Here's how the part is built. I have some questions about the finished solid (model axes, mm). Face numbers are marked on the shaded views. A direction names the side the tool comes from. Coordinates: 2 decimals unless noted, no trailing zeros. Write each loop counter-clockwise with the first axis right and the second up, starting at its lowest first coordinate (ties: lowest second). Pieces come first, ordered by that corner, then holes. Notation, with made-up numbers: (34.25, -2.5) - (76.25, -2.5) arc R23 ccw to (76.25, 14.5) - close; hole circle Ø5 at (-6.5, 58). An arc over 180 degrees is marked (long way). Answer in a Markdown table with one row per item. Add a question column.
Item 1: Imagine slicing it at B-B (y = 11). Please give me the cut outline in (x, z), plus the area to 3 significant figures.
Item 2: We'd pull the mould along Z, two halves only. Please class the marked faces 1, 2 and 3: +Z half, -Z half, draft (parallel to the pull), parting line (faces both ways), or undercut.
Item 3: If I drill on probe 1 along X at (y, z) = (12, 6); probe 2 along X at (y, z) = (10, 6); probe 3 along Y at (x, z) = (-8, 7.5), over which ranges is the centre line in solid material (lowest first)? Write a range as from..to.
Item 4: Imagine slicing it at D-D (z = 2.75). Please give me the cut outline in (x, y).
Item 5: I'm going to push flat-ended pins straight in: pin 1 (12 mm diameter, centred on x = -36, y = -3.5, fed in from -Z); pin 2 (5.5 mm diameter, centred on x = 1.95, z = 6, fed in from -Y); pin 3 (2 mm diameter, centred on x = -21, z = 8.5, fed in from -Y). Where does each tip first touch, or does it pass through?
Item 6: Imagine slicing it at C-C (x = -16). Please give me the cut outline in (y, z).
Item 7: Imagine slicing it at A-A (z = 10). Please give me the cut outline in (x, y), plus the area to 3 significant figures.
Item 8: Which directions (+Z, -Z, +X, -X, +Y, -Y) give clear straight access to the entire face, cutting with the end or side of a thin tool? Please do the marked faces 4 and 5.
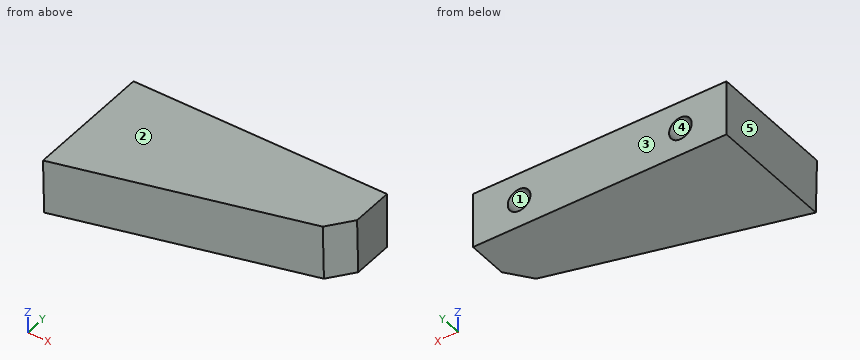
Autodesk Inventor part; units mm, degrees
ref_plane "作業平面8" through (7.9805, 5.1586, 3) normal (0.2539, -0.9668, -0.0285) x (-0.9522, -0.2551, 0.1679)
ref_plane "YZ Plane" through (0, 0, 0) normal (1, 0, 0) x (0, 1, 0)
ref_plane "XZ Plane" through (0, 0, 0) normal (0, 1, 0) x (-1, 0, 0)
sketch "スケッチ2" plane through (0, 0, 0) normal (0, 0, 1) x (1, 0, 0)
  line L0 (-43.0479, 19.0453) -> (-43.0479, -8.9547)
  line L1 (-43.0479, -8.9547) -> (11.9521, -8.9547)
  line L2 (11.9521, -8.9547) -> (11.9521, 19.0453)
  line L3 (11.9521, 19.0453) -> (-43.0479, 19.0453)
  point P0 (0, 0)
  dimension "d3" = 55
  dimension "d16" = 28
extrude "押し出し2" add sketch "スケッチ2" along normal blind 12
sketch "スケッチ4" plane through (-43.0479, 19.0453, 0) normal (0, 1, 0) x (1, 0, 0)
  line L0 (55, 0) -> (55, -12)
  line L1 (0, 0) -> (0, -12)
  line L2 (0, -6) -> (55, -6)
  line L3 (0, -12) -> (55, -12)
  line L4 (0, 0) -> (55, 0)
  point P0 (10, -6)
  point P1 (45, -6)
  dimension "d17" = 10
  dimension "d18" = 35
hole "穴2" at (-33.0479, 19.0453, 6) at (1.9521, 19.0453, 6) direction (0, -1, 0) diameter 4.917 depth 12 tip angle 118
ref_plane "作業平面8" through (7.9805, 5.1586, 3) normal (0.2539, -0.9668, -0.0285) x (-0.9522, -0.2551, 0.1679)
sketch "スケッチ7" plane through (7.9805, 5.1586, 3) normal (0.2539, -0.9668, -0.0285) x (-0.9522, -0.2551, 0.1679)
  line L0 (-7.2879, 16.2377) -> (59.5212, 16.2377)
  line L1 (59.5212, 16.2377) -> (59.5212, -15.7653)
  line L2 (59.5212, -15.7653) -> (-7.2879, -15.7653)
  line L3 (-7.2879, -15.7653) -> (-7.2879, 16.2377)
extrude "押し出し5" cut sketch "スケッチ7" along normal through all
chamfer "面取り1" distance 4 angle 45 1 edges at (11.9521, 6.1134, 6)
properties part number "100012" material "STEEL - HIGH GRADE ALLOY, BLACK OXIDE FINISH"
Here are the results:
| question | item | result |
|---|---|---|
| 1 | outline | (-43.05, 0) - (11.95, 0) - (11.95, 12) - (-43.05, 12) - close; hole circle Ø4.92 at (-33.05, 6); hole circle Ø4.92 at (1.95, 6) |
| 1 | area | 622 mm2 |
| 2 | face 1 | undercut |
| 2 | face 2 | +Z half |
| 2 | face 3 | draft |
| 3 | probe 1 | x = -43.05..-35.51, -30.59..-0.51, 4.41..11.95 |
| 3 | probe 2 | x = -43.05..-35.51, -30.59..-0.51, 4.41..11.86 |
| 3 | probe 3 | y = 0.83..19.05 |
| 4 | outline | (-43.05, -8.24) - (8.08, 5.19) - (11.95, 10.21) - (11.95, 19.05) - (-43.05, 19.05) - close |
| 5 | pin 1 | stops at z = 0 |
| 5 | pin 2 | stops at y = 2.76 |
| 5 | pin 3 | stops at y = -2.88 |
| 6 | outline | (-1.4, 12) - (-1.05, 0) - (19.05, 0) - (19.05, 12) - close |
| 7 | outline | (-43.05, -8.45) - (8.08, 4.98) - (11.95, 10) - (11.95, 19.05) - (-43.05, 19.05) - close |
| 7 | area | 1,110 mm2 |
| 8 | face 4 | +Y |
| 8 | face 5 | +Z, -Z, -X, +Y, -Y |
